```python
from build123d import *

# Parameters (mm, degrees)
BOSS_EXTRUDE2_DEPTH      = 22
BOSS_EXTRUDE2_DEPTH_BACK = 1
SKETCH2_W                = 20.249570214
SKETCH2_H                = 13.731042716
CUT_EXTRUDE1_DEPTH       = 43
SKETCH3_R                = 1.034515854
CUT_EXTRUDE2_DEPTH       = 43


with BuildPart() as part:
    # Sketch1 → Boss-Extrude2 (new, two sides: drawn at the far end of the back side and taken through both)
    with BuildSketch(Plane.XY.offset(-BOSS_EXTRUDE2_DEPTH_BACK)):
        Polygon((0, 0), (0, 15), (40, 15), align=None)
    extrude(amount=BOSS_EXTRUDE2_DEPTH + BOSS_EXTRUDE2_DEPTH_BACK)

    # Sketch2 → Cut-Extrude1 (cut)
    with BuildSketch(Plane.ZY):
        with Locations((10.512392638, 6.669693265)):
            Rectangle(SKETCH2_W, SKETCH2_H)
    extrude(amount=-CUT_EXTRUDE1_DEPTH, mode=Mode.SUBTRACT)

    # Sketch3 → Cut-Extrude2 (cut)
    with BuildSketch(Plane.XY.offset(22)):
        with Locations((2.111496697, 2.521392454)):
            Circle(SKETCH3_R)
    extrude(amount=-CUT_EXTRUDE2_DEPTH, mode=Mode.SUBTRACT)


solid = part.part
```
Can you work these out from the model? Positions are in its coordinate system, mm. A direction names the side the tool comes from. Give positions to 0.01 mm unless a question says otherwise; leave off trailing zeros. Write each loop counter-clockwise with the first axis right and the second up, starting at its lowest first coordinate (ties: lowest second). Pieces come first, ordered by that corner, then holes. Notation, with made-up numbers: (-21, 44) -> (-1, 44) arc R29 cw to (-1, 69) -> close; hole circle Ø3 at (30, 39). An arc over 180 degrees is marked (long way). Write item = value, one per line.
(1) Suppose I cut it at B-B on y = 7.25. Write out the boundary of the cut face in (x, z).
Worked out:
outline = (0, -1) -> (19.33, -1) -> (19.33, 0.39) -> (0, 0.39) -> close; (0, 20.64) -> (19.33, 20.64) -> (19.33, 22) -> (0, 22) -> close
(2) I need wall thicknesses on probe 1 along Z at (x, y) = (17, 8); probe 2 along Y at (x, z) = (17.5, 3.5); probe 3 along Y at (x, z) = (25.5, 21.25). Which ranges of each line are inside material? Lowest first, please. Write a range as from..to.
Worked out:
probe_1 = -1..0.39, 20.64..22
probe_2 = 13.54..15
probe_3 = 9.56..15
(3) For faces 4 (the face through (2.67, 3.39, 21.33)), 5 (the face through (18, 13.535, 10)), which set-ups out of +Z, -Z, +X, -X, +Y, -Y let a thin tool reach every point of the face, with its end or its side?
Worked out:
face_4 = +Z, -Z
face_5 = +X, -X, -Y
(4) I'm going to push a flat-ended pin straight in: P1, Ø4, axis at x = 24.5, z = 13.5, coming from the -Y side. Where does the tip first touch, or does it pass through?
Worked out:
P1 = 13.54
(5) Suppose I cut it at C-C on x = 24. Write out the boundary of the cut face in (y, z), then the cut area to 3 significant figures.
Worked out:
outline = (9, -1) -> (15, -1) -> (15, 22) -> (9, 22) -> (9, 20.64) -> (13.54, 20.64) -> (13.54, 0.39) -> (9, 0.39) -> close
area = 46.2 mm^2
(6) Thinking about a two-plate mould opening in Z: for faces 1 (the face through (10, 10, 0.388)), 2 (the face through (0, 14, 10)), 3 (the face through (11, 11, -1)), which applies, released by +Z, released by -Z, zero draft, split by the parting line, or undercut?
Worked out:
face_1 = undercut
face_2 = zero draft
face_3 = released by -Z
(7) Suppose I cut it at A-A on x = 30. Write out the boundary of the cut face in (y, z), then the cut area to 3 significant figures.
Worked out:
outline = (11.25, -1) -> (15, -1) -> (15, 22) -> (11.25, 22) -> (11.25, 20.64) -> (13.54, 20.64) -> (13.54, 0.39) -> (11.25, 0.39) -> close
area = 40.0 mm^2
(8) Suppose I cut it at D-D on z = 16.75. Write out the boundary of the cut face in (x, y).
Worked out:
outline = (0, 13.54) -> (36.09, 13.54) -> (40, 15) -> (0, 15) -> close
